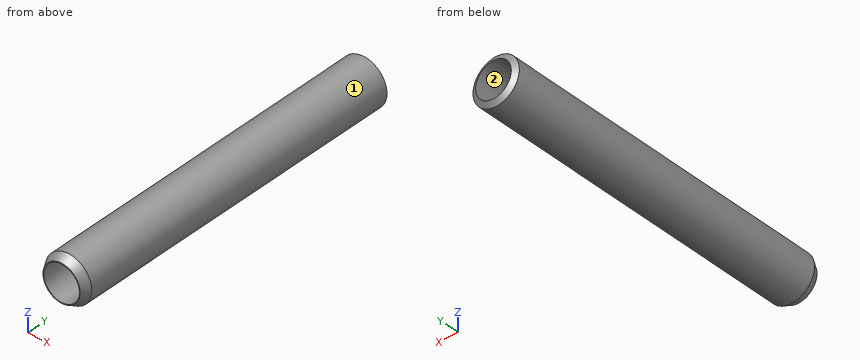
from build123d import *

# Parameters (mm, degrees)
SKETCH1_R           = 15
BOSS_EXTRUDE1_DEPTH = 224.642859
SKETCH2_R           = 11.538325124
CUT_EXTRUDE1_DEPTH  = 226.642225879
CHAMFER1_SIZE       = 2.968248
CHAMFER1_SIZE_2     = 5.183772


with BuildPart() as part:
    # Sketch1 → Boss-Extrude1 (new body)
    with BuildSketch(Plane(origin=(0, 0, 0), x_dir=(1, 0, 0), z_dir=(0, 1, 0))):
        with Locations(Location((0, 0, 0), (0, 0, 90))):
            Circle(SKETCH1_R)
    extrude(amount=BOSS_EXTRUDE1_DEPTH)

    # Sketch2 → Cut-Extrude1 (cut, through all)
    with BuildSketch(Plane(origin=(0, 0, 0), x_dir=(1, 0, 0), z_dir=(0, 1, 0))):
        with Locations(Location((0, 0, 0), (0, 0, 90))):
            Circle(SKETCH2_R)
    extrude(amount=CUT_EXTRUDE1_DEPTH, mode=Mode.SUBTRACT)

    # Chamfer1
    # the kernel refuses this chamfer: 5.183772, 2.968248 mm, written as the material it takes off along each edge
    with BuildSketch(Plane(origin=(0, 224.642859, 0), x_dir=(0, 0, -1), z_dir=(1, 0, 0))) as chamfer1_piece_1:
        Polygon((15, -CHAMFER1_SIZE), (15 - CHAMFER1_SIZE_2, 0), (15, 0), align=None)
    revolve(axis=Axis((0, 224.642859, 0), (0, 1, 0)), mode=Mode.SUBTRACT)
    with BuildSketch(Plane(origin=(0, 0, 0), x_dir=(0, 0, -1), z_dir=(1, 0, 0))) as chamfer1_piece_2:
        Polygon((15, CHAMFER1_SIZE_2), (15 - CHAMFER1_SIZE, 0), (15, 0), align=None)
    revolve(axis=Axis((0, 0, 0), (0, 1, 0)), mode=Mode.SUBTRACT)


solid = part.part
For this review, take the finished solid that the model builds, in its own axes (mm). Face numbers are marked on the shaded views. Coordinates: 2 decimals unless noted, no trailing zeros. Loops run counter-clockwise (first coordinate to the right, second up) from the corner with the lowest first, then second, coordinate; pieces in that order, holes last. Notation, with made-up numbers: (76, -25) - (128, -25) arc R15 cw to (128, -18) - close; hole circle Ø10 at (69, 29). An arc over 180 degrees is marked (long way). Use a Markdown table: item, result. Add a question column.
Item 1: Mouldability with a two-part tool opening along Z and no side actions: class the marked faces 1 and 2 as pulls with the +Z half, pulls with the -Z half, needs draft (parallel to the pull), parting line crosses it, or undercut.
Item 2: For line 1 (X direction, y = 71.5, z = 0); line 2 (X direction, y = 65.5, z = 4.5); line 3 (Z direction, x = -8.25, y = 21.5), list the stretches that pass through material, from the lowest coordinate up.
Item 3: We need section B-B (z = 0). Give the boundary of the cut face in (x, y), and give its area (3 significant figures).
Item 4: We need section C-C (y = 45). Give the boundary of the cut face in (x, z), and give its area (3 significant figures).
Item 5: Insertion check: pin 1 Ø3 at (x, y) = (-6, 116.5) entering from +Z; pin 2 Ø1.5 at (y, z) = (87.5, 4.5) entering from +X; pin 3 Ø12 at (y, z) = (102.5, -8) entering from +X. Each pin has a flat end and moves straight along its axis. Give the tip position at first contact, or say it passes through.
Item 6: We need section A-A (x = 0). Give the boundary of the cut face in (y, z), and give its area (3 significant figures).
Results list:
| question | item | result |
|---|---|---|
| 1 | face 1 | parting line crosses it |
| 1 | face 2 | undercut |
| 2 | line 1 | x = -15 to -11.54, 11.54 to 15 |
| 2 | line 2 | x = -14.31 to -10.62, 10.62 to 14.31 |
| 2 | line 3 | z = -12.53 to -8.07, 8.07 to 12.53 |
| 3 | outline | (-15, 5.18) - (-12.03, 0) - (-11.54, 0) - (-11.54, 223.66) - (-15, 221.67) - close; (11.54, 0) - (12.03, 0) - (15, 5.18) - (15, 221.67) - (11.54, 223.66) - close |
| 3 | area | 1,530 mm^2 |
| 4 | outline | circle Ø30 at (0, 0); hole circle Ø23.08 at (0, 0) |
| 4 | area | 289 mm^2 |
| 5 | pin 1 | stops at z = 14.31 |
| 5 | pin 2 | stops at x = 14.52 |
| 5 | pin 3 | stops at x = 14.87 |
| 6 | outline | (0, -12.03) - (5.18, -15) - (221.67, -15) - (223.66, -11.54) - (0, -11.54) - close; (0, 11.54) - (223.66, 11.54) - (221.67, 15) - (5.18, 15) - (0, 12.03) - close |
| 6 | area | 1,530 mm^2 |
